```python
from build123d import *

# Parameters (mm, degrees)
BOSS_EXTRUDE1_DEPTH        = 30.48
SKETCH2_W                  = 1.14
SKETCH2_H                  = 1.14
BOSS_EXTRUDE2_DEPTH        = 17.5
CHAMFER1_SIZE              = 0.25
CHAMFER2_SIZE              = 0.25
LPATTERN3_COUNT            = 6
LPATTERN3_PITCH            = 5.08
CHAMFER1_OF_LPATTERN3_SIZE = 0.25
CHAMFER2_OF_LPATTERN3_SIZE = 0.25


with BuildPart() as part:
    # Sketch1 → Boss-Extrude1 (new body)
    with BuildSketch(Plane(origin=(0, 0, 0), x_dir=(0, 0, -1), z_dir=(1, 0, 0))):
        with BuildLine():
            Line((0, 2.7), (0, 0.5))
            ThreePointArc((0, 0.5), (0.146446609, 0.146446609), (0.5, 0))
            Line((0.5, 0), (3.633974596, 0))
            ThreePointArc((3.633974596, 0), (3.883974596, 0.066987298), (4.066987298, 0.25))
            Line((4.066987298, 0.25), (4.5, 1))
            Line((4.5, 1), (6.5, 1))
            Line((6.5, 1), (7.050915041, 0.213211782))
            ThreePointArc((7.050915041, 0.213211782), (7.229616757, 0.056494583), (7.460491063, 0))
            Line((7.460491063, 0), (8.7, 0))
            ThreePointArc((8.7, 0), (9.760660172, 0.439339828), (10.2, 1.5))
            Line((10.2, 1.5), (10.2, 12.5))
            ThreePointArc((10.2, 12.5), (10.053553391, 12.853553391), (9.7, 13))
            Line((9.7, 13), (9.2, 13))
            ThreePointArc((9.2, 13), (8.846446609, 12.853553391), (8.7, 12.5))
            Line((8.7, 12.5), (8.7, 10.760283525))
            ThreePointArc((8.7, 10.760283525), (8.643505417, 10.529409219), (8.486788218, 10.350707503))
            Line((8.486788218, 10.350707503), (7.413211782, 9.59898119))
            ThreePointArc((7.413211782, 9.59898119), (7.256494583, 9.420279474), (7.2, 9.189405167))
            Line((7.2, 9.189405167), (7.2, 8.810594833))
            ThreePointArc((7.2, 8.810594833), (7.256494583, 8.579720526), (7.413211782, 8.40101881))
            Line((7.413211782, 8.40101881), (8.486788218, 7.649292497))
            ThreePointArc((8.486788218, 7.649292497), (8.643505417, 7.470590781), (8.7, 7.239716475))
            Line((8.7, 7.239716475), (8.7, 4.2))
            ThreePointArc((8.7, 4.2), (8.407106781, 3.492893219), (7.7, 3.2))
            Line((7.7, 3.2), (0.5, 3.2))
            ThreePointArc((0.5, 3.2), (0.146446609, 3.053553391), (0, 2.7))
        make_face()
    extrude(amount=BOSS_EXTRUDE1_DEPTH)

    # Sketch2 → Boss-Extrude2 (add)
    with BuildSketch(Plane(origin=(0, -3, 0), x_dir=(-1, 0, 0), z_dir=(0, -1, 0))):
        with Locations((-27.94, 5.5)):
            Rectangle(SKETCH2_W, SKETCH2_H)
    boss_extrude2 = extrude(amount=-BOSS_EXTRUDE2_DEPTH)

    # Chamfer1
    chamfer1_edges = [part.edges().sort_by_distance(p)[0] for p in [
        (27.37, -3, -5.5),
        (27.94, -3, -6.07),
        (28.51, -3, -5.5),
        (27.94, -3, -4.93),
    ]]
    chamfer(chamfer1_edges, length=CHAMFER1_SIZE)

    # Chamfer2
    chamfer2_edges = [part.edges().sort_by_distance(p)[0] for p in [
        (27.37, 14.5, -5.5),
        (27.94, 14.5, -4.93),
        (28.51, 14.5, -5.5),
        (27.94, 14.5, -6.07),
    ]]
    chamfer(chamfer2_edges, length=CHAMFER2_SIZE)

    # LPattern3: Boss-Extrude2 ×6
    with Locations(*[(-i * LPATTERN3_PITCH, 0, 0) for i in range(1, LPATTERN3_COUNT)]):
        add(boss_extrude2)

    # Chamfer1 of LPattern3
    chamfer1_of_lpattern3_edges = [part.edges().sort_by_distance(p)[0] for p in [
        (22.29, -3, -5.5),
        (22.86, -3, -6.07),
        (23.43, -3, -5.5),
        (22.86, -3, -4.93),
        (17.21, -3, -5.5),
        (17.78, -3, -6.07),
        (18.35, -3, -5.5),
        (17.78, -3, -4.93),
        (12.13, -3, -5.5),
        (12.7, -3, -6.07),
        (13.27, -3, -5.5),
        (12.7, -3, -4.93),
        (7.05, -3, -5.5),
        (7.62, -3, -6.07),
        (8.19, -3, -5.5),
        (7.62, -3, -4.93),
        (1.97, -3, -5.5),
        (2.54, -3, -6.07),
        (3.11, -3, -5.5),
        (2.54, -3, -4.93),
    ]]
    chamfer(chamfer1_of_lpattern3_edges, length=CHAMFER1_OF_LPATTERN3_SIZE)

    # Chamfer2 of LPattern3
    chamfer2_of_lpattern3_edges = [part.edges().sort_by_distance(p)[0] for p in [
        (22.29, 14.5, -5.5),
        (22.86, 14.5, -4.93),
        (23.43, 14.5, -5.5),
        (22.86, 14.5, -6.07),
        (17.21, 14.5, -5.5),
        (17.78, 14.5, -4.93),
        (18.35, 14.5, -5.5),
        (17.78, 14.5, -6.07),
        (12.13, 14.5, -5.5),
        (12.7, 14.5, -4.93),
        (13.27, 14.5, -5.5),
        (12.7, 14.5, -6.07),
        (7.05, 14.5, -5.5),
        (7.62, 14.5, -4.93),
        (8.19, 14.5, -5.5),
        (7.62, 14.5, -6.07),
        (1.97, 14.5, -5.5),
        (2.54, 14.5, -4.93),
        (3.11, 14.5, -5.5),
        (2.54, 14.5, -6.07),
    ]]
    chamfer(chamfer2_of_lpattern3_edges, length=CHAMFER2_OF_LPATTERN3_SIZE)


solid = part.part
```
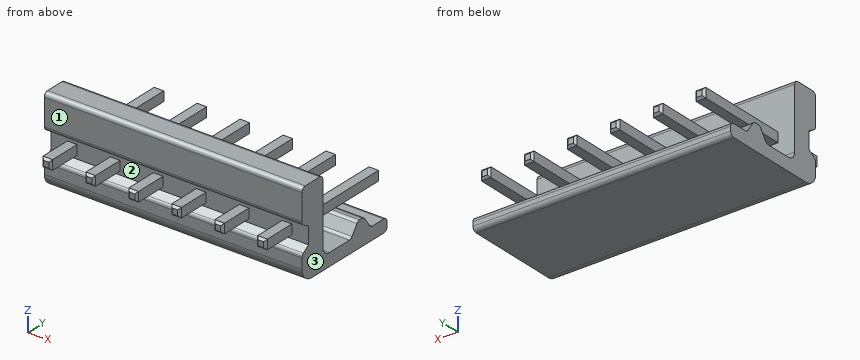
Could you check a few things on this model? Use its own coordinates, in mm. Face numbers are marked on the shaded views. Round coordinates to 2 decimals unless told otherwise and drop trailing zeros. Loops run counter-clockwise (first coordinate to the right, second up) from the corner with the lowest first, then second, coordinate; pieces in that order, holes last. Notation, with made-up numbers: (87, -23) - (101, -23) arc R25 cw to (101, -11) - close; hole circle Ø9 at (56.25, 67.25). An arc over 180 degrees is marked (long way). Answer as CSV lines item,"result".
1. Please list where these lines run through material, in increasing order: line 1 along X through (y, z) = (10, -5.5); line 2 along Z through (x, y) = (27.5, 10.75); line 3 along Z through (x, y) = (13, 8.75). Write a range as [from, to].
Filled in:
line 1,"x = [1.97, 3.11], [7.05, 8.19], [12.13, 13.27], [17.21, 18.35], [22.29, 23.43], [27.37, 28.51]"
line 2,"z = [-10.2, -8.7], [-6.07, -4.93]"
line 3,"z = [-10.2, -7.2], [-6.07, -4.93]"
2. I want a section at B-B on y = 5.75. List the corners of the cut face in (x, z) for me, then the cut area to 3 significant figures.
Filled in:
outline,"(0, -10.2) - (30.48, -10.2) - (30.48, -8.7) - (0, -8.7) - close; (1.97, -6.07) - (3.11, -6.07) - (3.11, -4.93) - (1.97, -4.93) - close; (7.05, -6.07) - (8.19, -6.07) - (8.19, -4.93) - (7.05, -4.93) - close; (12.13, -6.07) - (13.27, -6.07) - (13.27, -4.93) - (12.13, -4.93) - close; (17.21, -6.07) - (18.35, -6.07) - (18.35, -4.93) - (17.21, -4.93) - close; (22.29, -6.07) - (23.43, -6.07) - (23.43, -4.93) - (22.29, -4.93) - close; (27.37, -6.07) - (28.51, -6.07) - (28.51, -4.93) - (27.37, -4.93) - close"
area,"53.5 mm^2"
3. We'd pull the mould along X, two halves only. Please class the marked faces 1, 2 and 3: +X half, -X half, draft (parallel to the pull), parting line (faces both ways), or undercut.
Filled in:
face 1,"draft"
face 2,"undercut"
face 3,"+X half"
4. For pin 1 Ø0.9 at (y, z) = (9.5, -5.5) entering from -X; pin 2 Ø0.6 at (x, y) = (23, -0.5) entering from -Z; pin 3 Ø2 at (x, z) = (6, -1) entering from -Y; pin 4 Ø1.5 at (y, z) = (8, -3.5) entering from +X, each with a flat end and sliding along its axis, tell me the tip position at first contact or that it passes through.
Filled in:
pin 1,"stops at x = 1.97"
pin 2,"stops at z = -6.07"
pin 3,"stops at y = 0"
pin 4,"passes through"
5. I want a section at D-D on z = -3. List the corners of the cut face in (x, y) for me.
Filled in:
outline,"(0, 0) - (30.48, 0) - (30.48, 3.2) - (0, 3.2) - close"
6. I want a section at C-C on x = 6. List the corners of the cut face in (y, z) for me.
Filled in:
outline,"(0, -8.7) arc R1.5 ccw to (1.5, -10.2) - (12.5, -10.2) arc R0.5 ccw to (13, -9.7) - (13, -9.2) arc R0.5 ccw to (12.5, -8.7) - (10.76, -8.7) arc R0.5 cw to (10.35, -8.49) - (9.6, -7.41) arc R0.5 ccw to (9.19, -7.2) - (8.81, -7.2) arc R0.5 ccw to (8.4, -7.41) - (7.65, -8.49) arc R0.5 cw to (7.24, -8.7) - (4.2, -8.7) arc R1 cw to (3.2, -7.7) - (3.2, -0.5) arc R0.5 ccw to (2.7, 0) - (0.5, 0) arc R0.5 ccw to (0, -0.5) - (0, -3.63) arc R0.5 ccw to (0.25, -4.07) - (1, -4.5) - (1, -6.5) - (0.21, -7.05) arc R0.5 ccw to (0, -7.46) - close"
7. I want a section at A-A on y = -1.25. List the corners of the cut face in (x, z) for me, then the cut area to 3 significant figures.
Filled in:
outline,"(1.97, -6.07) - (3.11, -6.07) - (3.11, -4.93) - (1.97, -4.93) - close; (7.05, -6.07) - (8.19, -6.07) - (8.19, -4.93) - (7.05, -4.93) - close; (12.13, -6.07) - (13.27, -6.07) - (13.27, -4.93) - (12.13, -4.93) - close; (17.21, -6.07) - (18.35, -6.07) - (18.35, -4.93) - (17.21, -4.93) - close; (22.29, -6.07) - (23.43, -6.07) - (23.43, -4.93) - (22.29, -4.93) - close; (27.37, -6.07) - (28.51, -6.07) - (28.51, -4.93) - (27.37, -4.93) - close"
area,"7.80 mm^2"
